Model file for the job. Use its own axes, mm. Give positions to 0.01 mm unless a question says otherwise; leave off trailing zeros. Write each loop counter-clockwise with the first axis right and the second up, starting at its lowest first coordinate (ties: lowest second). Pieces come first, ordered by that corner, then holes. Notation, with made-up numbers: (79.5, 41.5) - (88.5, 41.5) arc R22 ccw to (88.5, 66.5) - close; hole circle Ø1 at (-24.5, 66). An arc over 180 degrees is marked (long way). Use a Markdown table: item, result. Add a question column.
Autodesk Inventor part; units mm, degrees
ref_plane "Start Plane" through (0, 0, -4.4541) normal (0, 0, 1) x (1, 0, 0)
ref_plane "End Plane" through (0, 0, 305.8974) normal (0, 0, 1) x (1, 0, 0)
ref_plane "Work Plane4" through (10.249, -2.9606, -4.8357) normal (-0.3966, 0.1146, -0.9108) x (-0.7636, 0.5095, 0.3966)
ref_plane "Start Plane" through (0, 0, -4.4541) normal (0, 0, 1) x (1, 0, 0)
ref_plane "End Plane" through (0, 0, 305.8974) normal (0, 0, 1) x (1, 0, 0)
sketch "Sketch" plane through (0, 0, 0) normal (0, 0, 1) x (1, 0, 0)
  circle A0 centre (0, 0) radius 6.9342
  circle A1 centre (0, 0) radius 10.668
  dimension "d0" = 21.336
  dimension "d1" = 3.7338
extrude "Body" add sketch "Sketch" along normal up to surface (310.3515 mm away) from surface at -4.4541
sketch "Sketch3" plane through (0, 0, 0) normal (0, 0, 1) x (1, 0, 0)
  line L0 (0, 0) -> (10, 0)
ref_plane "Work Plane3" through (0, 0, 0) normal (0, -1, 0) x (1, 0, 0)
sketch "Sketch4" plane through (0, 0, 0) normal (0, -1, 0) x (1, 0, 0)
  line L0 (-2, -4.4541) -> (12, -4.4541)
  line L1 (-2, 305.8974) -> (12, 305.8974)
  dimension "d7" = 310.3515
ref_plane "Work Plane4" through (10.249, -2.9606, -4.8357) normal (-0.3966, 0.1146, -0.9108) x (-0.7636, 0.5095, 0.3966)
split "Split1" plane through (10.249, -2.9606, -4.8357) removes the side toward (-0.3966, 0.1146, -0.9108)
ref_plane "Work Plane5" through (10.0091, 3.6912, -24.7602) normal (-0.8617, -0.3178, -0.3957) x (-0.2286, -0.4531, 0.8617)
split "Split2" plane through (10.0091, 3.6912, -24.7602) removes the side toward (-0.8617, -0.3178, -0.3957)
ref_plane "Work Plane6" through (-2.5393, -10.3614, -10.4394) normal (0.1665, 0.6793, -0.7147) x (0.9028, -0.3964, -0.1665)
split "Split3" plane through (-2.5393, -10.3614, -10.4394) removes the side toward (0.1665, 0.6793, -0.7147)
ref_plane "Work Plane7" through (-10.0742, -3.5095, 321.3152) normal (0.7992, 0.2784, 0.5327) x (0.5832, -0.1452, -0.7992)
split "Split4" plane through (-10.0742, -3.5095, 321.3152) removes the side toward (0.7992, 0.2784, 0.5327)
ref_plane "Work Plane8" through (10.668, 0, 310.6897) normal (-0.51, 0, 0.8602) x (0.8602, 0, 0.51)
split "Split5" plane through (10.668, 0, 310.6897) removes the side toward (-0.51, 0, 0.8602)
ref_plane "Work Plane9" through (-36.1517, -17.3472, 323.6752) normal (0.1548, -0.8989, 0.4098) x (0.8658, -0.0763, -0.4945)
sketch "Sketch5" plane through (-36.1517, -17.3472, 323.6752) normal (0.1548, -0.8989, 0.4098) x (0.8658, -0.0763, -0.4945)
  circle A0 centre (41.0585, -4.6699) radius 3
  point P0 (190.0204, -223.4181)
hole "Hole1" at (-2.823, -22.4951, 299.7942) direction (-0.1548, 0.8989, -0.4098) diameter 6 depth 25.4 tip angle 118
equation "\"d0\" = G_H"
equation "\"d1\" = G_T"
equation "\"d2\" = G_L"
equation "\"G_H\" = 21.336"
equation "\"G_T\" = 3.7338"
equation "\"G_L\" = 310.3515"
equation "\"G_OFFSET_START\" = 4.45413"
equation "\"G_OFFSET_END\" = 1.53222"
equation "\"d4\" = -G_OFFSET_START"
equation "\"d5\" = G_OFFSET_END + B_L"
equation "\"B_L\" = 304.36515"
properties part number "ANSI - 1/2 x 0.147 - 12.219" material "Steel, Mild"
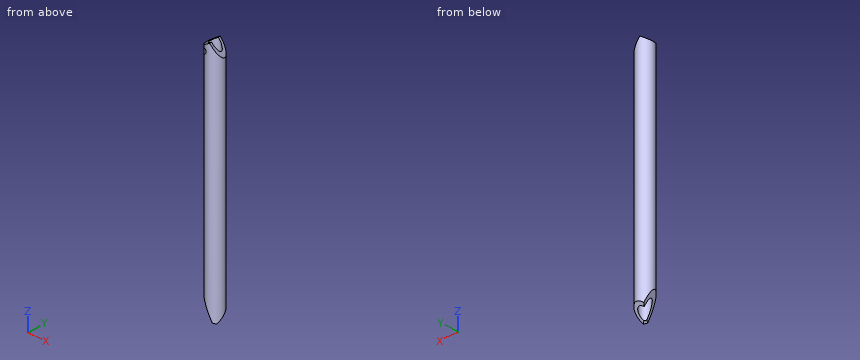
(1) Band-saw the part on A-A (z = 230). Write the cut outline in (x, y).
(2) Flat gauge pins, fed straight in: pin 1 (2 mm diameter, centred on y = -5, z = 77.5, fed in from +X); pin 2 (4 mm diameter, centred on x = 6, y = -1, fed in from +Z); pin 3 (4 mm diameter, centred on x = -5.5, z = 37, fed in from +Y). Where does each tip first touch, or does it go through?
(3) Probe probe 1 along Y at (x, z) = (0, 125.5); probe 2 along Z at (x, y) = (-7.5, -3.5). List the from-to ranges inside material, lowest first. Write a range as [from, to].
Model answer:
| question | item | result |
|---|---|---|
| 1 | outline | circle Ø21.34 at (0, 0); hole circle Ø13.87 at (0, 0) |
| 2 | pin 1 | stops at x = 9.89 |
| 2 | pin 2 | stops at z = 296.53 |
| 2 | pin 3 | stops at y = 10.08 |
| 3 | probe 1 | y = [-10.67, -6.93], [6.93, 10.67] |
| 3 | probe 2 | z = [19.14, 288.11], [293.94, 299.92] |
